```python
from build123d import *

# Parameters (mm, degrees)
SKETCH_1_R          = 1.25
EXTRUDE_1_DEPTH     = 145
CUT_EXTRUDE_1_DEPTH = 6
SKETCH_4_R          = 1.75
EXTRUDE_3_DEPTH     = 2
EXTRUDE_3_TAPER     = 64


with BuildPart() as part:
    # Эскиз1 → Бобышка-Вытянуть1 (new body)
    with BuildSketch(Plane(origin=(0, 0, 0), x_dir=(1, 0, 0), z_dir=(0, 1, 0))):
        with Locations(Location((0, 0, 0), (0, 0, 270))):
            Circle(SKETCH_1_R)
    extrude(amount=EXTRUDE_1_DEPTH)

    # Эскиз3 → Вырез-Вытянуть1 (cut, symmetric)
    with BuildSketch(Plane(origin=(0, 0, 0), x_dir=(0, 0, -1), z_dir=(1, 0, 0))):
        Polygon((1.25, 0), (-2.080626709, 0.599874475), (-2.080626709, 0), align=None)
    extrude(amount=CUT_EXTRUDE_1_DEPTH, both=True, mode=Mode.SUBTRACT)

    # Эскиз4 → Бобышка-Вытянуть3 (add)
    with BuildSketch(Plane(origin=(0, 0.218062, -0.039274839), x_dir=(1, 0, 0), z_dir=(0, -0.9841646858615077, 0.177256512159977))):
        with Locations((0, 0.040379775)):
            Circle(SKETCH_4_R)
    extrude(amount=EXTRUDE_3_DEPTH, taper=EXTRUDE_3_TAPER)


solid = part.part
```
The model under review builds one solid part; all positions refer to its coordinate system, in mm. A direction names the side the tool comes from. Give positions to 0.01 mm unless a question says otherwise; leave off trailing zeros. Loops run counter-clockwise (first coordinate to the right, second up) from the corner with the lowest first, then second, coordinate; pieces in that order, holes last. Notation, with made-up numbers: (70.5, -36) -> (82.5, -36) arc R20 cw to (82.5, -23) -> close; hole circle Ø5 at (-28, 85). An arc over 180 degrees is marked (long way). Use CSV: the item, a comma, the result in double quotes.
1. Machinability: for faces 1 (the face through (-1.22, 71.48, -0.27)), 2 (the face through (0, 145, 0)), which of the approach directions +Z, -Z, +X, -X, +Y, -Y give a long, thin tool a straight path to every point of the face, cutting with its end or side? Answer none if there is none.
Result:
face 1,"+Y"
face 2,"+Z, -Z, +X, -X, +Y"
2. For P1, Ø2, axis at y = 121.5, z = 0.5, coming from the +X side; P2, Ø2, axis at y = 45, z = -1.5, coming from the -X side, all flat-tipped, find the tip position at first contact; note any pin that passes through.
Result:
P1,"stops at x = 1.25"
P2,"stops at x = -1.15"
3. Consider section A-A, the plane y = 97.5. Write out the cut boundary in (x, z).
Result:
outline,"circle Ø2.5 at (0, 0)"
4. To check wall thickness, follow probe 1 along Z at (x, y) = (-0.1, 64); probe 2 along X at (y, z) = (12, -0.25); probe 3 along Y at (x, z) = (0, 1.2). State the ranges of each line that lie inside material, in increasing order. Write a range as from..to.
Result:
probe 1,"z = -1.25..1.25"
probe 2,"x = -1.22..1.22"
probe 3,"y = 0.15..145"
